The model under review builds one solid part; all positions refer to its coordinate system, in mm. A direction names the side the tool comes from. Round coordinates to 2 decimals unless told otherwise and drop trailing zeros. Order: outer loops, then holes, each group sorted by start corner. A loop starts at its lowest first (then second) coordinate and runs counter-clockwise, first axis right, second up. Notation, with made-up numbers: M 55.5,-9.75 L 96.5,-9.75 A26 ccw 96.5,15.25 Z; hole C 73,54.5 d6. An arc over 180 degrees is marked long. Use a Markdown table: item, result. Add a question column.
1. For faces 1 (the flat face through (110.89, 31.27, -4.93)), 2 (the flat face through (256.249, 166.376, -4.93)), 3 (the flat face through (58.702, 168.704, -4.93)), list the 3-axis set-ups (+Z, -Z, +X, -X, +Y, -Y) from which the entire face can be reached by the end or side of a thin tool; tool diameter is ignored.
2. Consider section C-C on y = 35.5. State the section outline as (x, z) points.
3. Insertion check: P1, Ø4, axis at x = 247.5, z = -6, coming from the -Y side; P2, Ø5, axis at y = 169, z = -8.5, coming from the +X side; P3, Ø2, axis at y = 220, z = -4, coming from the -X side. Each pin has a flat end and moves straight along its axis. Give the tip position at first contact, or say it passes through.
4. Consider section B-B on z = -8. State the section outline as (x, y) points.
5. Consider section D-D on y = 110. State the section outline as (x, z) points, then the cut area to 3 significant figures.
6. The part is to be moulded in two halves that separate along X. For faces 4 (the flat face through (220.309, 32.708, -4.93)), 5 (the flat face through (155, 173, -10)), 6 (the flat face through (210.1, 242.08, -4.93)), say which applies: +X half, -X half, draft (parallel to the pull), parting line (faces both ways), or undercut.
7. To check wall thickness, follow probe 1 along Y at (x, z) = (110.5, -2); probe 2 along Y at (x, z) = (219, -6); probe 3 along X at (y, z) = (209, -7.5). State the ranges of each line that lie inside material, in increasing order.
8. Consider section A-A on x = 214. State the section outline as (y, z) points.
from build123d import *

# Parameters (mm, degrees)
PAD_DEPTH = 10


with BuildPart() as part:
    # Sketch → Pad (new body)
    with BuildSketch(Plane.XY):
        Polygon((-38.693619, 95.521584), (-117.703079, 32.091431), (-224.532791, 32.091431), (-105.462189, -63.61018), (-180.020416, -183.79361), (-45.370419, -120.363464), (38.090302, -182.680801), (-25.339891, -55.820522), (90.392357, 22.076147), (9.157263, 22.076147), align=None)
    extrude(amount=-PAD_DEPTH)


with BuildPart() as part_1:
    # Body placement: moved
    add(part.part.moved(Location((224.532791, 183.79361, 0))))


solid = part_1.part
Answer block:
| question | item | result |
|---|---|---|
| 1 | face 1 | +Z, -Z, -Y |
| 1 | face 2 | +Z, -Z, +X |
| 1 | face 3 | +Z, -Z, -X |
| 2 | outline | M 66.54,-10 L 119.87,-10 L 119.87,0 L 66.54,0 Z; M 216.57,-10 L 245.43,-10 L 245.43,0 L 216.57,0 Z |
| 3 | P1 | y = 10.91 |
| 3 | P2 | x = 263.86 |
| 3 | P3 | x = 110.71 |
| 4 | outline | M 0,215.89 L 119.07,120.18 L 44.51,0 L 179.16,63.43 L 262.62,1.11 L 199.19,127.97 L 314.93,205.87 L 233.69,205.87 L 185.84,279.32 L 106.83,215.89 Z |
| 5 | outline | M 112.75,-10 L 208.18,-10 L 208.18,0 L 112.75,0 Z |
| 5 | area | 954 mm^2 |
| 6 | face 4 | undercut |
| 6 | face 5 | draft |
| 6 | face 6 | +X half |
| 7 | probe 1 | 31.09 to 106.37, 127.07 to 218.83 |
| 7 | probe 2 | 33.68 to 88.36, 141.3 to 228.42 |
| 7 | probe 3 | 8.57 to 231.65 |
| 8 | outline | M 37.42,-10 L 98.36,-10 L 98.36,0 L 37.42,0 Z; M 137.94,-10 L 236.09,-10 L 236.09,0 L 137.94,0 Z |
